Geometry: final body of the model. Coordinates: model frame, mm. Face numbers are marked on the shaded views. A direction names the side the tool comes from. Round coordinates to 2 decimals unless told otherwise and drop trailing zeros. Loops run counter-clockwise (first coordinate to the right, second up) from the corner with the lowest first, then second, coordinate; pieces in that order, holes last. Notation, with made-up numbers: (84.25, 34.25) - (119.25, 34.25) arc R10 cw to (119.25, 42.25) - close; hole circle Ø5 at (54, 13). An arc over 180 degrees is marked (long way). Answer as a JSON object with one key per item and string values. Group by question number.
Item 1: Section C-C (x = -13). Return the cut outline in (y, z) (3 decimals), plus the area to 3 significant figures.
Item 2: First-contact query: pin 1 (3.5 mm diameter, centred on x = -1.5, y = 0, fed in from -Z); pin 2 (0.6 mm diameter, centred on x = -15, y = -5, fed in from -Z); pin 3 (3 mm diameter, centred on x = 12.5, z = 3, fed in from +Y). Flat tips, straight axial feed; report the tip coordinate or a pass-through.
Item 3: Section B-B (z = 8). Return the cut outline in (x, y), plus the area to 3 significant figures.
Item 4: Reachability of the marked faces 1, 2, 3 and 4 from +Z, -Z, +X, -X, +Y, -Y: full face, straight path, thin tool, end or side. Return the list, or none.
Item 5: Draft query along Y for the marked faces 5, 6 and 7. Return one class per face: released by +Y, released by -Y, zero draft, split by the parting line, or undercut.
Item 6: Line query: line 1 (Y direction, x = -13, z = 0.9) (3 decimals); line 2 (Y direction, x = 12, z = 0.5); line 3 (Y direction, x = 0, z = 0.6). Output: solid intervals per line, ascending.
Item 7: Section A-A (y = 0). Return the cut outline in (x, z), plus the area to 3 significant figures.
```python
from build123d import *

# Parameters (mm, degrees)
BOSS_EXTRUDE1_DEPTH     = 2
SKETCH2_R               = 1.51
BOSS_EXTRUDE2_DEPTH     = 4
SKETCH3_R               = 3.5
BOSS_EXTRUDE3_DEPTH     = 1
SKETCH4_W               = 2
SKETCH4_H               = 17
BOSS_EXTRUDE4_DEPTH     = 0.001
SKETCH5_W               = 18
SKETCH5_H               = 2
BOSS_EXTRUDE5_DEPTH     = 0.001
SKETCH6_W               = 2.001
SKETCH6_H               = 2
BOSS_EXTRUDE6_DEPTH     = 5
BOSS_EXTRUDE7_DEPTH     = 0.001
CUT_EXTRUDE1_DEPTH      = 20.519323784
SKETCH9_W               = 2.937742252
SKETCH9_H               = 8
CUT_EXTRUDE2_DEPTH      = 0.001
CUT_EXTRUDE11_START     = -0.001
SKETCH21_R              = 9.75
SKETCH21_R_2            = 3.5
CUT_EXTRUDE11_DEPTH     = 0.001
SKETCH10_W              = 32
SKETCH10_H              = 2
BOSS_EXTRUDE8_DEPTH     = 7
FILLET1_R               = 0.5
SKETCH11_R              = 0.625
BOSS_EXTRUDE9_DEPTH     = 2
SKETCH14_W              = 2
SKETCH14_H              = 2
CUT_EXTRUDE5_DEPTH      = 22.401355237
SKETCH12_R              = 0.675
CUT_EXTRUDE3_DEPTH      = 2.5
CUT_EXTRUDE6_DEPTH      = 2
FILLET2_R               = 0.5
FILLET3_R               = 0.5
FILLET4_R               = 2
CUT_EXTRUDE7_DEPTH      = 26.019992106
CUT_EXTRUDE7_DEPTH_BACK = 1
SKETCH19_R              = 0.625
CUT_EXTRUDE9_DEPTH      = 2


with BuildPart() as part:
    # Sketch1 → Boss-Extrude1 (new body)
    with BuildSketch(Plane.XY):
        Polygon((-11, 6), (-11, 11), (11, 11), (11, 6), (11, -6), (-11, -6), align=None)
    extrude(amount=BOSS_EXTRUDE1_DEPTH)

    # Sketch3 → Boss-Extrude3 (add)
    with BuildSketch(Plane(origin=(0, 0, 0), x_dir=(-1, 0, 0), z_dir=(0, 0, -1))):
        with Locations(Location((0, 0, 0), (0, 0, 180))):
            Circle(SKETCH3_R)
    extrude(amount=BOSS_EXTRUDE3_DEPTH)

    # Sketch4 → Boss-Extrude4 (add)
    with BuildSketch(Plane(origin=(0, 0, 0), x_dir=(-1, 0, 0), z_dir=(0, 0, -1))):
        with Locations((10, 2.5)):
            Rectangle(SKETCH4_W, SKETCH4_H)
        with Locations((-10, 2.5)):
            Rectangle(SKETCH4_W, SKETCH4_H)
    extrude(amount=BOSS_EXTRUDE4_DEPTH)

    # Sketch5 → Boss-Extrude5 (add)
    with BuildSketch(Plane(origin=(0, 0, 0), x_dir=(-1, 0, 0), z_dir=(0, 0, -1))):
        with Locations((0, 10)):
            Rectangle(SKETCH5_W, SKETCH5_H)
    extrude(amount=BOSS_EXTRUDE5_DEPTH)

    # Sketch6 → Boss-Extrude6 (add)
    with BuildSketch(Plane(origin=(11, 0, 0), x_dir=(0, 0, -1), z_dir=(1, 0, 0))):
        with Locations((-0.9995, -5)):
            Rectangle(SKETCH6_W, SKETCH6_H)
        with Locations((-0.9995, 5)):
            Rectangle(SKETCH6_W, SKETCH6_H)
    boss_extrude6 = extrude(amount=BOSS_EXTRUDE6_DEPTH)

    # Mirror1: Boss-Extrude6 across plane
    add(boss_extrude6.mirror(Plane(origin=(0, 0, 0), x_dir=(0, 0, 1), z_dir=(1, 0, 0))))

    # Sketch7 → Boss-Extrude7 (add)
    with BuildSketch(Plane(origin=(0, 0, -0.001), x_dir=(-1, 0, 0), z_dir=(0, 0, -1))):
        with BuildLine():
            ThreePointArc((-6.708203932, -6), (-8.407551231, -3.211398808), (-9, 0))
            Line((-9, 0), (-9, -6))
            Line((-9, -6), (-6.708203932, -6))
        make_face()
        with BuildLine():
            Line((-9, 9), (-9, 0))
            ThreePointArc((-9, 0), (-6.363961031, 6.363961031), (0, 9))
            Line((0, 9), (-9, 9))
        make_face()
    boss_extrude7 = extrude(amount=-BOSS_EXTRUDE7_DEPTH)

    # Sketch8 → Cut-Extrude1 (cut, through all)
    with BuildSketch(Plane(origin=(0, 0, -0.001), x_dir=(-1, 0, 0), z_dir=(0, 0, -1))):
        with BuildLine():
            Line((-11, 4), (-9.16515139, 4))
            ThreePointArc((-9.16515139, 4), (-10, 0), (-9.16515139, -4))
            Line((-9.16515139, -4), (-11, -4))
            Line((-11, -4), (-11, 4))
        make_face()
    cut_extrude1 = extrude(amount=-CUT_EXTRUDE1_DEPTH, mode=Mode.SUBTRACT)

    # Sketch9 → Cut-Extrude2 (cut)
    with BuildSketch(Plane(origin=(0, 0, -0.001), x_dir=(-1, 0, 0), z_dir=(0, 0, -1))):
        with Locations((-9.531128874, 0)):
            Rectangle(SKETCH9_W, SKETCH9_H)
    cut_extrude2 = extrude(amount=-CUT_EXTRUDE2_DEPTH, mode=Mode.SUBTRACT)

    # Mirror2: Boss-Extrude7, Cut-Extrude1, Cut-Extrude2 across plane
    add(boss_extrude7.mirror(Plane(origin=(0, 0, 0), x_dir=(0, 0, 1), z_dir=(1, 0, 0))))
    add(cut_extrude1.mirror(Plane(origin=(0, 0, 0), x_dir=(0, 0, 1), z_dir=(1, 0, 0))), mode=Mode.SUBTRACT)
    add(cut_extrude2.mirror(Plane(origin=(0, 0, 0), x_dir=(0, 0, 1), z_dir=(1, 0, 0))), mode=Mode.SUBTRACT)

    # Sketch21 → Cut-Extrude11 (cut)
    with BuildSketch(Plane(origin=(0, 0, -0.001), x_dir=(-1, 0, 0), z_dir=(0, 0, -1)).offset(CUT_EXTRUDE11_START)):
        Circle(SKETCH21_R)
        with Locations(Location((0, 0, 0), (0, 0, 180))):
            Circle(SKETCH21_R_2, mode=Mode.SUBTRACT)
    extrude(amount=CUT_EXTRUDE11_DEPTH, mode=Mode.SUBTRACT)

    # Sketch10 → Boss-Extrude8 (add)
    with BuildSketch(Plane.XY.offset(2)):
        with Locations((0, -5)):
            Rectangle(SKETCH10_W, SKETCH10_H)
        with Locations((0, 5)):
            Rectangle(SKETCH10_W, SKETCH10_H)
    extrude(amount=BOSS_EXTRUDE8_DEPTH)

    # Fillet1
    fillet1_edges = [part.edges().sort_by_distance(p)[0] for p in [
        (10, 0, 2),
        (-10, 0, 2),
    ]]
    fillet(fillet1_edges, radius=FILLET1_R)

    # Sketch11 → Boss-Extrude9 (add)
    with BuildSketch(Plane(origin=(0, 0, -0.001), x_dir=(-1, 0, 0), z_dir=(0, 0, -1))):
        with Locations(Location((-13, -5, 0), (0, 0, 180))):
            Circle(SKETCH11_R)
    boss_extrude9 = extrude(amount=BOSS_EXTRUDE9_DEPTH)

    # Sketch14 → Cut-Extrude5 (cut, through all)
    with BuildSketch(Plane(origin=(0, 0, -0.001), x_dir=(-1, 0, 0), z_dir=(0, 0, -1))):
        with Locations((10, 7)):
            Rectangle(SKETCH14_W, SKETCH14_H)
        with Locations((-10, 7)):
            Rectangle(SKETCH14_W, SKETCH14_H)
    extrude(amount=-CUT_EXTRUDE5_DEPTH, mode=Mode.SUBTRACT)

    # Sketch12 → Cut-Extrude3 (cut)
    with BuildSketch(Plane(origin=(0, 0, -0.001), x_dir=(-1, 0, 0), z_dir=(0, 0, -1))):
        with Locations((13, -5)):
            Circle(SKETCH12_R)
    cut_extrude3 = extrude(amount=-CUT_EXTRUDE3_DEPTH, mode=Mode.SUBTRACT)

    # Sketch16 → Cut-Extrude6 (cut)
    with BuildSketch(Plane(origin=(0, 6, 0), x_dir=(1, 0, 0), z_dir=(0, 1, 0))):
        with BuildLine():
            Line((-9, -1), (-9, -2))
            ThreePointArc((-9, -2), (-8.75, -1.5), (-9, -1))
        make_face()
    cut_extrude6 = extrude(amount=CUT_EXTRUDE6_DEPTH, mode=Mode.SUBTRACT)

    # Mirror3: Boss-Extrude9, Cut-Extrude3 across plane
    add(boss_extrude9.mirror(Plane.ZX))
    add(cut_extrude3.mirror(Plane.ZX), mode=Mode.SUBTRACT)

    # Mirror4: Cut-Extrude6 across plane
    add(cut_extrude6.mirror(Plane(origin=(0, 0, 0), x_dir=(0, 0, 1), z_dir=(1, 0, 0))), mode=Mode.SUBTRACT)

    # Fillet2
    fillet2_edges = [part.edges().sort_by_distance(p)[0] for p in [
        (12.375, -5, -0.001),
        (12.375, 5, -0.001),
    ]]
    fillet(fillet2_edges, radius=FILLET2_R)

    # Fillet3
    # the kernel refuses this fillet: 0.5 mm, written as the material it takes off along each edge
    with BuildSketch(Plane(origin=(-13, -5, -0.001), x_dir=(-1, 0, 0), z_dir=(0, -1, 0))) as fillet3_piece_1:
        with BuildLine():
            CenterArc((0.675 + FILLET3_R, -FILLET3_R), FILLET3_R, 90, 90)
            Line((0.675, -FILLET3_R), (0.675, 0))
            Line((0.675, 0), (0.675 + FILLET3_R, 0))
        make_face()
    revolve(axis=Axis((-13, -5, -0.001), (0, 0, -1)), mode=Mode.SUBTRACT)
    with BuildSketch(Plane(origin=(-13, 5, -0.001), x_dir=(-1, 0, 0), z_dir=(0, 1, 0))) as fillet3_piece_2:
        with BuildLine():
            CenterArc((0.675 + FILLET3_R, FILLET3_R), FILLET3_R, 180, 90)
            Line((0.675, FILLET3_R), (0.675, 0))
            Line((0.675, 0), (0.675 + FILLET3_R, 0))
        make_face()
    revolve(axis=Axis((-13, 5, -0.001), (0, 0, 1)), mode=Mode.SUBTRACT)

    # Fillet4
    fillet4_edges = [part.edges().sort_by_distance(p)[0] for p in [
        (16, -5, 9),
        (-16, -5, 9),
        (-16, 5, 9),
        (16, 5, 9),
    ]]
    fillet(fillet4_edges, radius=FILLET4_R)

    # Sketch17 → Cut-Extrude7 (cut, two sides: drawn at the far end of the back side and taken through both)
    with BuildSketch(Plane.XZ.offset(6).offset(-CUT_EXTRUDE7_DEPTH_BACK)):
        with BuildLine():
            Line((-16, 7), (-16, -0.001))
            Line((-16, -0.001), (-14.5, -0.001))
            Line((-14.5, -0.001), (-14.5, 7))
            ThreePointArc((-14.5, 7), (-14.353553391, 7.353553391), (-14, 7.5))
            Line((-14, 7.5), (14, 7.5))
            ThreePointArc((14, 7.5), (14.353553391, 7.353553391), (14.5, 7))
            Line((14.5, 7), (14.5, -0.001))
            Line((14.5, -0.001), (16, -0.001))
            Line((16, -0.001), (16, 7))
            ThreePointArc((16, 7), (15.414213562, 8.414213562), (14, 9))
            Line((14, 9), (-14, 9))
            ThreePointArc((-14, 9), (-15.414213562, 8.414213562), (-16, 7))
        make_face()
    extrude(amount=CUT_EXTRUDE7_DEPTH + CUT_EXTRUDE7_DEPTH_BACK, mode=Mode.SUBTRACT)

    # Sketch19 → Cut-Extrude9 (cut)
    with BuildSketch(Plane(origin=(0, 6, 0), x_dir=(1, 0, 0), z_dir=(0, 1, 0))):
        with Locations(Location((0, -2.625, 0), (0, 0, 90))):
            Circle(SKETCH19_R)
        with Locations(Location((0, -8.125, 0), (0, 0, 270))):
            Circle(SKETCH19_R)
    extrude(amount=-CUT_EXTRUDE9_DEPTH, mode=Mode.SUBTRACT)


with BuildPart() as body_2:
    # Sketch2 → Boss-Extrude2 (new body)
    with BuildSketch(Plane(origin=(0, 0, 2), x_dir=(-1, 0, 0), z_dir=(0, 0, -1))):
        Circle(SKETCH2_R)
    extrude(amount=BOSS_EXTRUDE2_DEPTH)


with BuildPart() as part_1:
    add(part.part)

    # Combine2: cut body 2
    add(body_2.part, mode=Mode.SUBTRACT)


solid = part_1.part
```
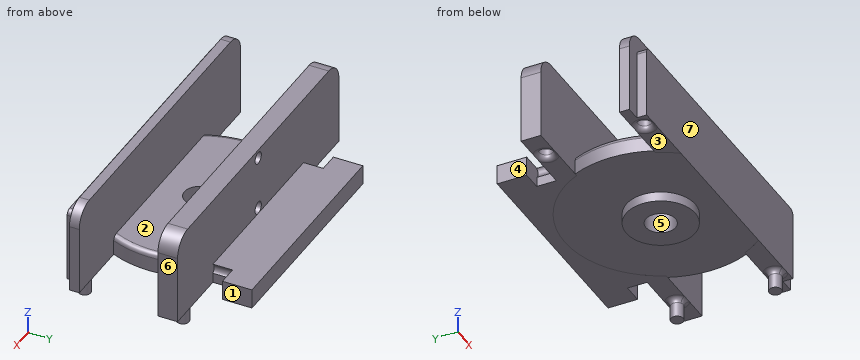
Values:
{
 "1": {"outline": "(-6, 0.031) arc R0.5 ccw to (-5.675, 0.499) - (-5.675, 2.499) - (-4.325, 2.499) - (-4.325, 0.499) arc R0.5 ccw to (-4, 0.031) - (-4, 9) - (-5, 9) - (-5, 7.5) - (-6, 7.5) - close; (4, 0.031) arc R0.5 ccw to (4.325, 0.499) - (4.325, 2.499) - (5.675, 2.499) - (5.675, 0.499) arc R0.5 ccw to (6, 0.031) - (6, 9) - (4, 9) - close", "area": "27.5 mm^2"},
 "2": {"pin 1": "stops at z = -1", "pin 2": "stops at z = 0", "pin 3": "stops at y = 6"},
 "3": {"outline": "(-15.73, -5) - (15.73, -5) - (15.73, -4) - (-15.73, -4) - close; (-15.73, 4) - (-0.61, 4) - (-0.61, 6) - (-15.73, 6) - close; (0.61, 4) - (15.73, 4) - (15.73, 6) - (0.61, 6) - close", "area": "91.9 mm^2"},
 "4": {"face 1": "+Z, -Z, +X, +Y", "face 2": "+Z, +X, -X", "face 3": "-Z, -X, +Y, -Y", "face 4": "+Z, -Z, -X, +Y"},
 "5": {"face 5": "undercut", "face 6": "zero draft", "face 7": "released by -Y"},
 "6": {"line 1": "y = -6 to -5.675, -4.325 to -4, 4 to 4.325, 5.675 to 6", "line 2": "y = -6 to -4, 4 to 6", "line 3": "y = -6 to -1.51, 1.51 to 11"},
 "7": {"outline": "(-10, 0) - (-3.5, 0) - (-3.5, -1) - (-1.51, -1) - (-1.51, 2) - (-9.5, 2) arc R0.5 ccw to (-10, 1.5) - close; (1.51, -1) - (3.5, -1) - (3.5, 0) - (10, 0) - (10, 1.5) arc R0.5 ccw to (9.5, 2) - (1.51, 2) - close", "area": "37.8 mm^2"}
}
